from build123d import *

# Parameters (mm, degrees)
F1_DEPTH  = 0.762
F2_R      = 1.905
F4_DEPTH  = 19.05
F5_R      = 1.905
F7_DEPTH  = 25.4
F8_R      = 1.905
F11_R     = 3.175
F11_R_2   = 1.27
F12_DEPTH = 5.334
F13_DEPTH = 2.54


with BuildPart() as f1:
    # F0 (on Top) → F1 (new body)
    with BuildSketch(Plane.XY):
        Polygon((19.05, 32.995568), (-19.05, 32.995568), (-38.1, 0), (-19.05, -32.995568), (19.05, -32.995568), (38.1, 0), align=None)
    extrude(amount=F1_DEPTH)

    # F2
    f2_edges = [f1.edges().sort_by_distance(p)[0] for p in [
        (38.1, 0, 0.381),
        (19.05, 32.995568, 0.381),
        (-19.05, 32.995568, 0.381),
        (-38.1, 0, 0.381),
        (-19.05, -32.995568, 0.381),
        (19.05, -32.995568, 0.381),
    ]]
    fillet(f2_edges, radius=F2_R)



with BuildPart() as f4:
    # F3 (on Top) → F4 (new body)
    with BuildSketch(Plane.XY):
        Polygon((18.415, 31.895716), (-18.415, 31.895716), (-36.83, 0), (-18.415, -31.895716), (18.415, -31.895716), (36.83, 0), align=None)
    extrude(amount=F4_DEPTH)

    # F5
    f5_edges = [f4.edges().sort_by_distance(p)[0] for p in [
        (-18.415, -31.895716, 9.525),
        (18.415, -31.895716, 9.525),
        (36.83, 0, 9.525),
        (-36.83, 0, 9.525),
        (18.415, 31.895716, 9.525),
        (-18.415, 31.895716, 9.525),
    ]]
    fillet(f5_edges, radius=F5_R)


with BuildPart() as f7:
    # F6 (on Top) → F7 (new body)
    with BuildSketch(Plane.XY):
        Polygon((17.907, 31.015834), (-17.907, 31.015834), (-35.814, 0), (-17.907, -31.015834), (17.907, -31.015834), (35.814, 0), align=None)
    extrude(amount=F7_DEPTH)

    # F8
    f8_edges = [f7.edges().sort_by_distance(p)[0] for p in [
        (-17.907, -31.015834, 12.7),
        (17.907, -31.015834, 12.7),
        (35.814, 0, 12.7),
        (-35.814, 0, 12.7),
        (17.907, 31.015834, 12.7),
        (-17.907, 31.015834, 12.7),
    ]]
    fillet(f8_edges, radius=F8_R)


with BuildPart() as f7_1:
    # F9: moved
    add(f7.part.moved(Location((0, 0, 0.762))))


with BuildPart() as f4_1:
    add(f4.part)

    # F10: cut F7
    add(f7_1.part, mode=Mode.SUBTRACT)


with BuildPart() as f1_1:
    add(f1.part)

    add(f4_1.part)  # F12 merges F4
    # F11 (on face) → F12 (join)
    with BuildSketch(Plane.XY.offset(0.762)):
        with Locations((-9.2075, 15.875)):
            Circle(F11_R)
        with Locations((-9.2075, 15.875)):
            Circle(F11_R_2, mode=Mode.SUBTRACT)
        with Locations((9.2075, 15.875)):
            Circle(F11_R)
        with Locations((9.2075, 15.875)):
            Circle(F11_R_2, mode=Mode.SUBTRACT)
        with Locations((9.2075, -15.875)):
            Circle(F11_R)
        with Locations((9.2075, -15.875)):
            Circle(F11_R_2, mode=Mode.SUBTRACT)
        with Locations((-9.2075, -15.875)):
            Circle(F11_R)
        with Locations((-9.2075, -15.875)):
            Circle(F11_R_2, mode=Mode.SUBTRACT)
    extrude(amount=F12_DEPTH)

    # F11 (on face) → F13 (cut)
    with BuildSketch(Plane.XY.offset(0.762)):
        Polygon((-1.099852, 11.84275), (1.099852, 11.84275), (2.199705, 13.74775), (1.099852, 15.65275), (-1.099852, 15.65275), (-2.199705, 13.74775), align=None)
    extrude(amount=-F13_DEPTH, mode=Mode.SUBTRACT)


solid = f1_1.part
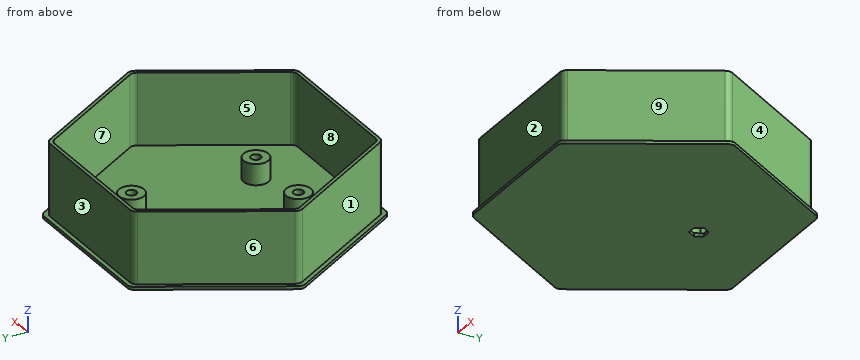
Input: part model. Units: mm. Frame: model coordinates. Face numbers are marked on the shaded views. A direction names the side the tool comes from. Round coordinates to 2 decimals unless told otherwise and drop trailing zeros. Loops run counter-clockwise (first coordinate to the right, second up) from the corner with the lowest first, then second, coordinate; pieces in that order, holes last. Notation, with made-up numbers: (51.25, 44) -> (60.25, 44) arc R25 cw to (60.25, 58) -> close; hole circle Ø6 at (21, 10). An arc over 180 degrees is marked (long way). Answer as a JSON object with one key per item and string values. Group by question number.
1) Pin query (flat end, axial travel): pin 1 (7 mm diameter, centred on x = -9.5, y = 15.5, fed in from +Z); pin 2 (1.5 mm diameter, centred on x = 9.21, y = 15.88, fed in from +Z); pin 3 (4 mm diameter, centred on y = 11, z = 5, fed in from +X). Return the tip coordinate at first contact, or that it passes through.
2) Section query A-A on z = 3. State how many separate pieces and enclosed holes the cut face has, plus the area to 3 significant figures.
3) Ray query, L1, parallel to Y at x = -4.5, z = 10.5; L2, parallel to Z at x = -1.5, y = 6; L3, parallel to X at y = -12.5, z = 6.5. Return the intervals inside material, ascending.
4) Section query C-C on y = 11. Output: boundary loops of the cut face in (x, z), plus the area to 3 significant figures.
5) Section query D-D on x = -33. Output: boundary loops of the cut face in (y, z).
6) Draft query along X for the marked faces 6, 7, 8 and 9. Return one class per face: +X half, -X half, draft (parallel to the pull), parting line (faces both ways), or undercut.
7) Reachability of the marked faces 1, 2, 3, 4 and 5 from +Z, -Z, +X, -X, +Y, -Y: full face, straight path, thin tool, end or side. Return the list, or none.
8) Section query B-B on z = 13. Output: boundary loops of the cut face in (x, y) (1 decimal).
Reply:
{
 "1": {"pin 1": "stops at z = 6.1", "pin 2": "stops at z = 0.76", "pin 3": "stops at x = 31.63"},
 "2": {"separate pieces": "5", "enclosed holes": "5", "area": "298 mm2"},
 "3": {"L1": "y = -31.9 to -31.02, 31.02 to 31.9", "L2": "z = 0 to 0.76", "L3": "x = -29.61 to -28.6, 28.6 to 29.61"},
 "4": {"outline": "(-31.75, 0) -> (31.75, 0) -> (31.75, 0.76) -> (30.48, 0.76) -> (30.48, 19.05) -> (29.46, 19.05) -> (29.46, 0.76) -> (-29.46, 0.76) -> (-29.46, 19.05) -> (-30.48, 19.05) -> (-30.48, 0.76) -> (-31.75, 0.76) -> close", "area": "85.5 mm2"},
 "5": {"outline": "(-8.83, 0) -> (8.83, 0) -> (8.83, 0.76) -> (6.63, 0.76) -> (6.63, 19.05) -> (4.87, 19.05) -> (4.87, 0.76) -> (-4.87, 0.76) -> (-4.87, 19.05) -> (-6.63, 19.05) -> (-6.63, 0.76) -> (-8.83, 0.76) -> close"},
 "6": {"face 6": "-X half", "face 7": "undercut", "face 8": "undercut", "face 9": "+X half"},
 "7": {"face 1": "+Z, -X, -Y", "face 2": "+Z, +X, -X, -Y", "face 3": "+Z, +X, -X, +Y", "face 4": "+Z, +X, +Y", "face 5": "+Z"},
 "8": {"outline": "(-36.3, -1) -> (-19, -30.9) arc R1.9 ccw to (-17.3, -31.9) -> (17.3, -31.9) arc R1.9 ccw to (19, -30.9) -> (36.3, -1) arc R1.9 ccw to (36.3, 1) -> (19, 30.9) arc R1.9 ccw to (17.3, 31.9) -> (-17.3, 31.9) arc R1.9 ccw to (-19, 30.9) -> (-36.3, 1) arc R1.9 ccw to start; hole (-35.3, -1) -> (-18.5, -30.1) arc R1.9 ccw to (-16.8, -31) -> (16.8, -31) arc R1.9 ccw to (18.5, -30.1) -> (35.3, -1) arc R1.9 ccw to (35.3, 1) -> (18.5, 30.1) arc R1.9 ccw to (16.8, 31) -> (-16.8, 31) arc R1.9 ccw to (-18.5, 30.1) -> (-35.3, 1) arc R1.9 ccw to start"}
}
